Could you check a few things on this model? Use its own coordinates, in mm. Give positions to 0.01 mm unless a question says otherwise; leave off trailing zeros. Loops run counter-clockwise (first coordinate to the right, second up) from the corner with the lowest first, then second, coordinate; pieces in that order, holes last. Notation, with made-up numbers: (-0.75, -7.5) - (16.25, -7.5) arc R20 ccw to (16.25, 26.5) - close; hole circle Ø2 at (61.25, 44.5). An arc over 180 degrees is marked (long way). Write each question's results on one line, items separated by ' | '. Start each with the question number.
(1) Suppose I cut it at A-A (z = 2.5). Please give me the cut outline in (x, y), and give its area (3 significant figures).
(2) I need wall thicknesses on line 1 (Z direction, x = 0.5, y = 3.5); line 2 (X direction, y = 5, z = 2); line 3 (X direction, y = 3.25, z = -60). Which ranges of each line are inside material? Lowest first, please.
(3) For pin 1 (1.9 mm diameter, centred on y = 3.5, z = -16.5, fed in from +X); pin 2 (3 mm diameter, centred on x = -32.5, y = 4.5, fed in from -Z); pin 3 (1.9 mm diameter, centred on x = -130, y = 2.5, fed in from +Z), each with a flat end and sliding along its axis, tell me the tip position at first contact or that it passes through.
(4) Suppose I cut it at C-C (z = -39.5). Please give me the cut outline in (x, y), and give its area (3 significant figures).
(5) Suppose I cut it at B-B (x = -7). Please give me the cut outline in (y, z), and give its area (3 significant figures).
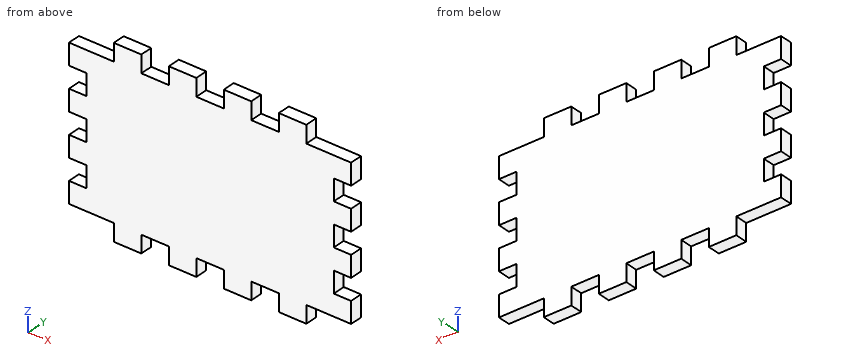
Autodesk Inventor part; units mm, degrees
ref_plane "YZ Plane" through (0, 0, 0) normal (1, 0, 0) x (0, 1, 0)
ref_plane "XZ Plane" through (0, 0, 0) normal (0, 1, 0) x (-1, 0, 0)
ref_plane "XY Plane" through (0, 0, 0) normal (0, 0, 1) x (1, 0, 0)
sketch "Sketch1" plane through (0, 0, 0) normal (0, 1, 0) x (-1, 0, 0)
  line L0 (0, 0) -> (127, 0)
  line L1 (127, 0) -> (127, -76.2)
  line L2 (127, -76.2) -> (0, -76.2)
  line L3 (0, -76.2) -> (0, 0)
  dimension "BoxHeight" = 127
  dimension "d1" = 76.2
sketch "Sketch2" plane through (0, 0, 0) normal (0, 1, 0) x (-1, 0, 0)
  line L0 (0, 0) -> (-8.89, 0)
  line L1 (-8.89, 0) -> (-8.89, -10.8857)
  line L2 (-8.89, -10.8857) -> (0, -10.8857)
  line L3 (0, -10.8857) -> (0, 0)
  line L4 (0, -76.2) -> (0, 0)
  line L5 (0, 0) -> (127, 0)
  line L6 (0, -21.7714) -> (-8.89, -21.7714)
  line L7 (-8.89, -21.7714) -> (-8.89, -32.6571)
  line L8 (-8.89, -32.6571) -> (0, -32.6571)
  line L9 (0, -32.6571) -> (0, -21.7714)
  line L10 (0, -43.5429) -> (-8.89, -43.5429)
  line L11 (-8.89, -43.5429) -> (-8.89, -54.4286)
  line L12 (-8.89, -54.4286) -> (0, -54.4286)
  line L13 (0, -54.4286) -> (0, -43.5429)
  line L14 (63.5, 0) -> (63.5, -115.824) construction
  line L15 (127, -10.8857) -> (127, 0)
  line L16 (127, -76.2) -> (127, 0)
  line L17 (127, -32.6571) -> (127, -21.7714)
  line L18 (127, -54.4286) -> (127, -43.5429)
  line L19 (28.2222, -76.2) -> (14.1111, -76.2)
  line L20 (14.1111, -76.2) -> (14.1111, -85.09)
  line L21 (14.1111, -85.09) -> (28.2222, -85.09)
  line L22 (28.2222, -85.09) -> (28.2222, -76.2)
  line L23 (127, -76.2) -> (0, -76.2)
  line L24 (56.4444, -76.2) -> (42.3333, -76.2)
  line L25 (42.3333, -76.2) -> (42.3333, -85.09)
  line L26 (42.3333, -85.09) -> (56.4444, -85.09)
  line L27 (56.4444, -85.09) -> (56.4444, -76.2)
  line L28 (84.6667, -76.2) -> (70.5556, -76.2)
  line L29 (70.5556, -76.2) -> (70.5556, -85.09)
  line L30 (70.5556, -85.09) -> (84.6667, -85.09)
  line L31 (84.6667, -85.09) -> (84.6667, -76.2)
  line L32 (112.8889, -76.2) -> (98.7778, -76.2)
  line L33 (98.7778, -76.2) -> (98.7778, -85.09)
  line L34 (98.7778, -85.09) -> (112.8889, -85.09)
  line L35 (112.8889, -85.09) -> (112.8889, -76.2)
  line L36 (127, -38.1) -> (0, -38.1) construction
  line L37 (63.5, -76.2) -> (63.5, 39.624) construction
  line L38 (28.2222, 0) -> (14.1111, 0)
  line L39 (14.1111, 0) -> (14.1111, 8.89)
  line L40 (14.1111, 8.89) -> (28.2222, 8.89)
  line L41 (28.2222, 8.89) -> (28.2222, 0)
  line L42 (127, 0) -> (0, 0)
  line L43 (56.4444, 0) -> (42.3333, 0)
  line L44 (42.3333, 0) -> (42.3333, 8.89)
  line L45 (42.3333, 8.89) -> (56.4444, 8.89)
  line L46 (56.4444, 8.89) -> (56.4444, 0)
  line L47 (84.6667, 0) -> (70.5556, 0)
  line L48 (70.5556, 0) -> (70.5556, 8.89)
  line L49 (84.6667, 8.89) -> (84.6667, 0)
  line L50 (70.5556, 8.89) -> (84.6667, 8.89)
  line L51 (112.8889, 0) -> (98.7778, 0)
  line L52 (98.7778, 0) -> (98.7778, 8.89)
  line L53 (112.8889, 8.89) -> (112.8889, 0)
  line L54 (98.7778, 8.89) -> (112.8889, 8.89)
  line L55 (0, -65.3143) -> (-8.89, -65.3143)
  line L56 (-8.89, -65.3143) -> (-8.89, -76.2)
  line L57 (-8.89, -76.2) -> (0, -76.2)
  line L58 (0, -76.2) -> (0, -65.3143)
  line L59 (127, 0) -> (135.89, 0)
  line L60 (135.89, 0) -> (135.89, -10.8857)
  line L61 (135.89, -10.8857) -> (127, -10.8857)
  line L62 (127, -10.8857) -> (127, 0)
  line L63 (127, -76.2) -> (127, 0)
  line L64 (127, -21.7714) -> (135.89, -21.7714)
  line L65 (135.89, -21.7714) -> (135.89, -32.6571)
  line L66 (135.89, -32.6571) -> (127, -32.6571)
  line L67 (127, -32.6571) -> (127, -21.7714)
  line L68 (127, -43.5429) -> (135.89, -43.5429)
  line L69 (135.89, -43.5429) -> (135.89, -54.4286)
  line L70 (135.89, -54.4286) -> (127, -54.4286)
  line L71 (127, -54.4286) -> (127, -43.5429)
  line L72 (135.89, -65.3143) -> (135.89, -76.2)
  line L73 (127, -65.3143) -> (135.89, -65.3143)
  line L74 (135.89, -76.2) -> (127, -76.2)
  line L75 (127, -76.2) -> (127, -65.3143)
  dimension "d2" = 8.89
  dimension "d3" = 10.8857
  dimension "d5" = 8.89
  dimension "d6" = 10.8857
  dimension "d7" = 10.8857
  dimension "d8" = 8.89
  dimension "d9" = 10.8857
  dimension "d10" = 10.8857
  dimension "d11" = 14.1111
  dimension "d12" = 127
  dimension "d13" = 14.1111
  dimension "d14" = 8.89
  dimension "d15" = 8.89
  dimension "d16" = 14.1111
  dimension "d17" = 8.89
  dimension "d18" = 14.1111
  dimension "d22" = 8.89
  dimension "d23" = 14.1111
  dimension "d27" = 14.1111
  dimension "d28" = 14.1111
  dimension "d29" = 14.1111
  dimension "d34" = 76.2
  dimension "d35" = 8.89
  dimension "d36" = 10.8857
  dimension "d41" = 10.8857
extrude "Connections" add sketch "Sketch2" along normal blind 6.35 contours L3 L2 L1 L0 | L39 L40 L41 L5 | L4 L8 L7 L6 | L44 L45 L46 L5 | L4 L12 L11 L10 | L48 L50 L49 L5 | L4 L57 L56 L55 | L52 L54 L53 L5 | L19 L22 L21 L20 | L59 L60 L61 L15 | L23 L27 L26 L25 | L64 L65 L66 L16 | L23 L31 L30 L29 | L68 L69 L70 L16 | L23 L35 L34 L33 | L73 L72 L74 L16
extrude "Base Extrusion" add sketch "Sketch1" along normal blind 6.35
sketch "Sketch3" plane through (0, 6.35, 0) normal (0, 1, 0) x (1, 0, 0)
  line L0 (-6.6713, 46.5048) -> (-6.6713, 27.1528) construction
  line L1 (-6.6713, 27.1528) -> (-46.955, 27.1528) construction
  line L2 (-46.955, 27.1528) -> (-46.955, 46.5048) construction
  line L3 (-46.955, 46.5048) -> (-6.6713, 46.5048) construction
  point P0 (0, 0)
sketch "Sketch4" plane through (0, 0, 0) normal (0, -1, 0) x (1, 0, 0)
  line L0 (-84.6667, 8.89) -> (-70.5556, 8.89)
  line L1 (-84.6667, 0) -> (-84.6667, 8.89)
  line L2 (-84.6667, 0) -> (-98.7778, 0)
  line L3 (-98.7778, 0) -> (-98.7778, 8.89)
  line L4 (-98.7778, 8.89) -> (-112.8889, 8.89)
  line L5 (-112.8889, 8.89) -> (-112.8889, 0)
  line L6 (-135.89, 0) -> (-112.8889, 0)
  line L7 (-135.89, -10.8857) -> (-135.89, 0)
  line L8 (-127, -10.8857) -> (-135.89, -10.8857)
  line L9 (-127, -10.8857) -> (-127, -21.7714)
  line L10 (-135.89, -21.7714) -> (-127, -21.7714)
  line L11 (-135.89, -32.6571) -> (-135.89, -21.7714)
  line L12 (-127, -32.6571) -> (-135.89, -32.6571)
  line L13 (-127, -32.6571) -> (-127, -43.5429)
  line L14 (-135.89, -43.5429) -> (-127, -43.5429)
  line L15 (-135.89, -54.4286) -> (-135.89, -43.5429)
  line L16 (-127, -54.4286) -> (-135.89, -54.4286)
  line L17 (-127, -54.4286) -> (-127, -65.3143)
  line L18 (-127, -65.3143) -> (-135.89, -65.3143)
  line L19 (-135.89, -65.3143) -> (-135.89, -76.2)
  line L20 (-135.89, -76.2) -> (-112.8889, -76.2)
  line L21 (-112.8889, -76.2) -> (-112.8889, -85.09)
  line L22 (-112.8889, -85.09) -> (-98.7778, -85.09)
  line L23 (-98.7778, -85.09) -> (-98.7778, -76.2)
  line L24 (-98.7778, -76.2) -> (-84.6667, -76.2)
  line L25 (-84.6667, -76.2) -> (-84.6667, -85.09)
  line L26 (-84.6667, -85.09) -> (-70.5556, -85.09)
  line L27 (-70.5556, -85.09) -> (-70.5556, -76.2)
  line L28 (-70.5556, -76.2) -> (-56.4444, -76.2)
  line L29 (-56.4444, -85.09) -> (-56.4444, -76.2)
  line L30 (-42.3333, -85.09) -> (-56.4444, -85.09)
  line L31 (-42.3333, -76.2) -> (-42.3333, -85.09)
  line L32 (-42.3333, -76.2) -> (-28.2222, -76.2)
  line L33 (-28.2222, -85.09) -> (-28.2222, -76.2)
  line L34 (-14.1111, -85.09) -> (-28.2222, -85.09)
  line L35 (-14.1111, -76.2) -> (-14.1111, -85.09)
  line L36 (-14.1111, -76.2) -> (8.89, -76.2)
  line L37 (8.89, -76.2) -> (8.89, -65.3143)
  line L38 (8.89, -65.3143) -> (0, -65.3143)
  line L39 (0, -65.3143) -> (0, -54.4286)
  line L40 (8.89, -54.4286) -> (0, -54.4286)
  line L41 (8.89, -43.5429) -> (8.89, -54.4286)
  line L42 (0, -43.5429) -> (8.89, -43.5429)
  line L43 (0, -43.5429) -> (0, -32.6571)
  line L44 (8.89, -32.6571) -> (0, -32.6571)
  line L45 (8.89, -21.7714) -> (8.89, -32.6571)
  line L46 (0, -21.7714) -> (8.89, -21.7714)
  line L47 (0, -21.7714) -> (0, -10.8857)
  line L48 (8.89, -10.8857) -> (0, -10.8857)
  line L49 (8.89, 0) -> (8.89, -10.8857)
  line L50 (-14.1111, 0) -> (8.89, 0)
  line L51 (-14.1111, 0) -> (-14.1111, 8.89)
  line L52 (-14.1111, 8.89) -> (-28.2222, 8.89)
  line L53 (-28.2222, 8.89) -> (-28.2222, 0)
  line L54 (-28.2222, 0) -> (-42.3333, 0)
  line L55 (-42.3333, 8.89) -> (-42.3333, 0)
  line L56 (-56.4444, 8.89) -> (-42.3333, 8.89)
  line L57 (-56.4444, 0) -> (-56.4444, 8.89)
  line L58 (-56.4444, 0) -> (-70.5556, 0)
  line L59 (-70.5556, 8.89) -> (-70.5556, 0)
  point P0 (0, 0)
equation "\"d1\" = BaseLength"
equation "\"d2\" = PerpA"
equation "\"d3\" = PerpB"
equation "\"d5\" = d2"
equation "\"d6\" = d3"
equation "\"d7\" = PerpSpace"
equation "\"d8\" = d2"
equation "\"d9\" = d3"
equation "\"d10\" = d7"
equation "\"d11\" = -0.8 * d13 + 0.2 * d12"
equation "\"d13\" = 0.111111 * d12"
equation "\"d14\" = WallConA"
equation "\"d15\" = d14"
equation "\"d16\" = d13"
equation "\"d17\" = d15"
equation "\"d18\" = d20"
equation "\"d22\" = d14"
equation "\"d23\" = d25"
equation "\"d27\" = d11"
equation "\"d28\" = d27"
equation "\"d29\" = d11"
equation "\"d35\" = d37"
equation "\"d36\" = d38"
equation "\"d41\" = d10"
equation "\"d20\" = 0.111111 * d21"
equation "\"d25\" = 0.111111 * d26"
equation "\"d37\" = d39"
equation "\"d38\" = d40"
properties part number "WallToWall(Perpendicular1)"
Output values:
1) outline: (-112.89, 0) - (-98.78, 0) - (-98.78, 6.35) - (-112.89, 6.35) - close; (-84.67, 0) - (-70.56, 0) - (-70.56, 6.35) - (-84.67, 6.35) - close; (-56.44, 0) - (-42.33, 0) - (-42.33, 6.35) - (-56.44, 6.35) - close; (-28.22, 0) - (-14.11, 0) - (-14.11, 6.35) - (-28.22, 6.35) - close | area: 358 mm2
2) line 1: -76.2 to -65.31, -54.43 to -43.54, -32.66 to -21.77, -10.89 to 0 | line 2: -112.89 to -98.78, -84.67 to -70.56, -56.44 to -42.33, -28.22 to -14.11 | line 3: -127 to 0
3) pin 1: x = 0 | pin 2: z = -76.2 | pin 3: z = 0
4) outline: (-127, 0) - (0, 0) - (0, 6.35) - (-127, 6.35) - close | area: 806 mm2
5) outline: (0, -76.2) - (6.35, -76.2) - (6.35, 0) - (0, 0) - close | area: 484 mm2
